```python
from build123d import *

# Parameters (mm, degrees)
SKETCH_W        = 110
SKETCH_H        = 80
PAD_DEPTH       = 50
SKETCH001_R     = 1.5
POCKET_DEPTH    = 48
FILLET_R        = 2
FILLET001_R     = 2
SKETCH002_R     = 2.55
SKETCH002_W     = 11.5
SKETCH002_H     = 19.1
POCKET001_DEPTH = 5
SKETCH003_R     = 2.55
POCKET002_DEPTH = 5
SKETCH004_R     = 4.5
SKETCH004_R_2   = 2.55
PAD001_DEPTH    = 0.5
SKETCH005_R     = 4.5
SKETCH005_R_2   = 2.55
PAD002_DEPTH    = 0.5


with BuildPart() as part:
    # Sketch → Pad (new body)
    with BuildSketch(Plane.XY):
        with Locations((55, 40)):
            Rectangle(SKETCH_W, SKETCH_H)
    extrude(amount=PAD_DEPTH)

    # Sketch001 (on Face6 of Pad) → Pocket (cut)
    with BuildSketch(Plane.XY.offset(50)):
        with Locations((6, 74)):
            Circle(SKETCH001_R)
        with Locations((104, 74)):
            Circle(SKETCH001_R)
        with Locations((104, 6)):
            Circle(SKETCH001_R)
        with Locations((6, 6)):
            Circle(SKETCH001_R)
        Polygon((2, 10), (10, 10), (10, 2), (100, 2), (100, 10), (108, 10), (108, 70), (100, 70), (100, 78), (10, 78), (10, 70), (2, 70), align=None)
    extrude(amount=-POCKET_DEPTH, mode=Mode.SUBTRACT)

    # Fillet
    fillet_edges = [part.edges().sort_by_distance(p)[0] for p in [
        (0, 80, 25),
        (0, 40, 0),
        (0, 0, 25),
        (55, 0, 0),
        (110, 0, 25),
        (110, 80, 25),
        (110, 40, 0),
        (55, 80, 0),
    ]]
    fillet(fillet_edges, radius=FILLET_R)

    # Fillet001
    fillet001_edges = [part.edges().sort_by_distance(p)[0] for p in [
        (100, 10, 26),
        (100, 70, 26),
        (10, 70, 26),
        (10, 10, 26),
    ]]
    fillet(fillet001_edges, radius=FILLET001_R)

    # Sketch002 (on Face22 of Fillet001) → Pocket001 (cut)
    with BuildSketch(Plane.YZ.offset(110)):
        with Locations((15, 27.5)):
            Circle(SKETCH002_R)
        with Locations((28.75, 27.5)):
            Rectangle(SKETCH002_W, SKETCH002_H)
    extrude(amount=-POCKET001_DEPTH, mode=Mode.SUBTRACT)

    # Sketch003 (on Face18 of Pocket001) → Pocket002 (cut)
    with BuildSketch(Plane.XZ):
        with Locations((90, 27.5)):
            Circle(SKETCH003_R)
    extrude(amount=-POCKET002_DEPTH, mode=Mode.SUBTRACT)

    # Sketch004 (on Face22 of Pocket002) → Pad001 (join)
    with BuildSketch(Plane.YZ.offset(110)):
        with Locations((15, 27.5)):
            Circle(SKETCH004_R)
        with Locations((15, 27.5)):
            Circle(SKETCH004_R_2, mode=Mode.SUBTRACT)
    extrude(amount=PAD001_DEPTH)

    # Sketch005 (on Face18 of Pad001) → Pad002 (join)
    with BuildSketch(Plane.XZ):
        with Locations((90, 27.5)):
            Circle(SKETCH005_R)
        with Locations((90, 27.5)):
            Circle(SKETCH005_R_2, mode=Mode.SUBTRACT)
    extrude(amount=PAD002_DEPTH)


solid = part.part
```
The model under review builds one solid part; all positions refer to its coordinate system, in mm. A direction names the side the tool comes from. Give positions to 0.01 mm unless a question says otherwise; leave off trailing zeros. Write each loop counter-clockwise with the first axis right and the second up, starting at its lowest first coordinate (ties: lowest second). Pieces come first, ordered by that corner, then holes.
(1) Consider section C-C, the plane z = 12.5. Give the boundary of the cut face in (x, y), and give its area (3 significant figures).
(2) Consider section D-D, the plane x = 6. Give the boundary of the cut face in (y, z), and give its area (3 significant figures).
(3) Consider section B-B, the plane y = 15. Give the boundary of the cut face in (x, z), and give its area (3 significant figures).
(4) For P1, Ø5, axis at x = 106, z = 29.5, coming from the -Y side; P2, Ø5, axis at y = 74.5, z = 28.5, coming from the +X side; P3, Ø1.6, axis at x = 109, z = 25.5, coming from the +Y side, all flat-tipped, find the tip position at first contact; note any pin that passes through.
(5) The part is to be moulded in two halves that separate along Y. For faces 1 (the flat face through (108, 40, 26)), 2 (the flat face through (54, 80, 26)), 3 (the cylindrical face through (85.504, -0.246, 27.698)), say which applies: released by +Y, released by -Y, zero draft, split by the parting line, or undercut.
(6) Tool access review of faces 4 (the flat face through (5, 70, 26)), 5 (the flat face through (54, 41, 0)): name each direction out of +Z, -Z, +X, -X, +Y, -Y from which nothing blocks a thin tool from reaching the whole face with its end or side.
(7) Consider section A-A, the plane x = 90. Give the boundary of the cut face in (y, z), and give its area (3 significant figures).
(8) To check wall thickness, follow L1, parallel to X at y = 74, z = 28; L2, parallel to X at y = 43, z = 37.5; L3, parallel to Y at x = 77.5, z = 20. State the ranges of each line that lie inside material, in increasing order.
Returned:
1. outline: (0, 2) arc R2 ccw to (2, 0) - (108, 0) arc R2 ccw to (110, 2) - (110, 78) arc R2 ccw to (108, 80) - (2, 80) arc R2 ccw to (0, 78) - close; hole (2, 10) - (8, 10) arc R2 cw to (10, 8) - (10, 2) - (100, 2) - (100, 8) arc R2 cw to (102, 10) - (108, 10) - (108, 70) - (102, 70) arc R2 cw to (100, 72) - (100, 78) - (10, 78) - (10, 72) arc R2 cw to (8, 70) - (2, 70) - close; hole circle Ø3 at (6, 6); hole circle Ø3 at (6, 74); hole circle Ø3 at (104, 6); hole circle Ø3 at (104, 74)
1. area: 965 mm2
2. outline: (0, 2) arc R2 ccw to (2, 0) - (78, 0) arc R2 ccw to (80, 2) - (80, 50) - (75.5, 50) - (75.5, 2) - (72.5, 2) - (72.5, 50) - (70, 50) - (70, 2) - (10, 2) - (10, 50) - (7.5, 50) - (7.5, 2) - (4.5, 2) - (4.5, 50) - (0, 50) - close
2. area: 830 mm2
3. outline: (0, 2) arc R2 ccw to (2, 0) - (108, 0) arc R2 ccw to (110, 2) - (110, 23) - (110.5, 23) - (110.5, 24.95) - (108, 24.95) - (108, 2) - (2, 2) - (2, 50) - (0, 50) - close; (108, 30.05) - (110.5, 30.05) - (110.5, 32) - (110, 32) - (110, 50) - (108, 50) - close
3. area: 402 mm2
4. P1: stops at y = 0
4. P2: stops at x = 110
4. P3: stops at y = 79.99
5. face 1: undercut
5. face 2: released by +Y
5. face 3: zero draft
6. face 4: +Z
6. face 5: -Z, +X, -X, +Y, -Y
7. outline: (-0.5, 23) - (0, 23) - (0, 2) arc R2 ccw to (2, 0) - (78, 0) arc R2 ccw to (80, 2) - (80, 50) - (78, 50) - (78, 2) - (2, 2) - (2, 24.95) - (-0.5, 24.95) - close; (-0.5, 30.05) - (2, 30.05) - (2, 50) - (0, 50) - (0, 32) - (-0.5, 32) - close
7. area: 342 mm2
8. L1: x = 0 to 4.5, 7.5 to 10, 100 to 102.5, 105.5 to 110
8. L2: x = 0 to 2, 108 to 110
8. L3: y = 0 to 2, 78 to 80
